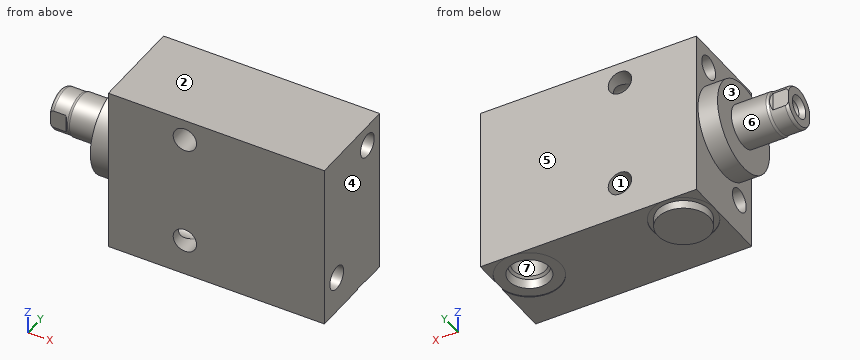
from build123d import *

# Parameters (mm, degrees)
SKETCH1_W          = 50.8
SKETCH1_H          = 28.575
EXTRUDE1_DEPTH     = 65.8368
SKETCH5_R          = 13.5001
EXTRUDE2_DEPTH     = 5.969
SKETCH6_W          = 6.35
SKETCH6_H          = 16.891
CUT_EXTRUDE4_DEPTH = 30.48
SKETCH13_R         = 7.874
EXTRUDE3_DEPTH     = 2.54
HOLE1_D            = 7.1374
HOLE1_DEPTH        = 65.8368
HOLE2_D            = 7.1374
HOLE2_DEPTH        = 28.575


with BuildPart() as part:
    # Sketch1 → Extrude1 (new body)
    with BuildSketch(Plane(origin=(0, 0, 0), x_dir=(0, 0, -1), z_dir=(1, 0, 0))):
        with Locations((2.3876, 0)):
            Rectangle(SKETCH1_W, SKETCH1_H)
    extrude(amount=EXTRUDE1_DEPTH)

    # S2D0002 → Cut-Revolve1 (revolve, cut)
    with BuildSketch(Plane(origin=(0, 4.7625, 0), x_dir=(-1, 0, 0), z_dir=(0, 1, 0)), mode=Mode.PRIVATE) as cut_revolve1_sk:
        Polygon((-15.7099, -27.5336), (-19.0499873, -27.5336), (-19.0499873, -27.7876), (-9.525, -27.7876), (-9.525, -13.5636), (-14.5034, -13.5636), (-14.5034, -24.316993135), (-15.167306865, -24.9809), align=None)
    revolve(cut_revolve1_sk.sketch.rotate(Axis((9.525, 4.7625, -19.13842003), (0, 0, 1)), 180), axis=Axis((9.525, 4.7625, -19.13842003), (0, 0, 1)), mode=Mode.SUBTRACT)  # turned: the seam where the file's is

    # Sketch3 → Cut-Revolve2 (revolve, cut)
    with BuildSketch(Plane(origin=(41.148, 4.7625, -25.146), x_dir=(1, 0, 0), z_dir=(0, 1, 0))):
        Polygon((21.5519, 2.3876), (24.8919873, 2.3876), (24.8919873, 2.6416), (15.367, 2.6416), (15.367, -11.5824), (20.3454, -11.5824), (20.3454, -0.829006865), (21.009306865, -0.1651), align=None)
    revolve(axis=Axis((56.515, 4.7625, -3.189624441), (0, 0, -1)), mode=Mode.SUBTRACT)

    # Sketch5 → Extrude2 (add)
    with BuildSketch(Plane.ZY):
        Circle(SKETCH5_R)
    extrude(amount=EXTRUDE2_DEPTH)

    # Sketch6 → Revolve1 (revolve)
    with BuildSketch(Plane(origin=(0, 0, 0), x_dir=(0, 0, 1), z_dir=(0, -1, 0)), mode=Mode.PRIVATE) as revolve1_sk:
        with Locations((-3.175, 14.4145)):
            Rectangle(SKETCH6_W, SKETCH6_H)
    revolve(revolve1_sk.sketch.rotate(Axis((5.754582971, 0, 0), (-1, 0, 0)), 180), axis=Axis((5.754582971, 0, 0), (-1, 0, 0)))  # turned: the seam where the file's is

    # S2D0001 → Cut-Revolve4 (revolve, cut)
    with BuildSketch(Plane(origin=(-18.511260017, 3.2639, 0), x_dir=(0, 1, 0), z_dir=(0, 0, 1)), mode=Mode.PRIVATE) as cut_revolve4_sk:
        Polygon((-0.7112, 2.786949769), (-0.7112, -11.653260017), (-3.2639, -13.18707692), (-3.2639, 4.348739983), (0.1905, 4.348739983), align=None)
    revolve(cut_revolve4_sk.sketch.rotate(Axis((0, 0, 0), (-1, 0, 0)), 90), axis=Axis((0, 0, 0), (-1, 0, 0)), mode=Mode.SUBTRACT)  # turned: the seam where the file's is

    # Sketch8 → Cut-Revolve5 (revolve, cut)
    with BuildSketch(Plane(origin=(0, 0, 0), x_dir=(0, 0, -1), z_dir=(0, 1, 0)), mode=Mode.PRIVATE) as cut_revolve5_sk:
        with BuildLine():
            Line((-6.35, 16.5354), (-6.096, 17.2974))
            Line((-6.096, 17.2974), (-6.096, 21.844))
            ThreePointArc((-6.096, 21.844), (-5.995678675, 22.387796865), (-5.707922533, 22.86))
            Line((-5.707922533, 22.86), (-6.35, 22.86))
            Line((-6.35, 22.86), (-6.35, 16.5354))
        make_face()
    revolve(cut_revolve5_sk.sketch.rotate(Axis((-12.65936, 0, 0), (-1, 0, 0)), 180), axis=Axis((-12.65936, 0, 0), (-1, 0, 0)), mode=Mode.SUBTRACT)  # turned: the seam where the file's is

    # Sketch12 → Cut-Extrude4 (cut, symmetric)
    with BuildSketch(Plane(origin=(0, 0, 0), x_dir=(0, -1, 0), z_dir=(0, 0, -1))):
        Polygon((5.461, 22.86), (5.461, 18.0848), (6.096, 17.4498), (6.096, 22.86), align=None)
        Polygon((-5.461, 22.86), (-5.461, 18.0848), (-6.096, 17.4498), (-6.096, 22.86), align=None)
    extrude(amount=CUT_EXTRUDE4_DEPTH, both=True, mode=Mode.SUBTRACT)

    # Sketch13 → Extrude3 (add)
    with BuildSketch(Plane(origin=(0, 0, -27.5336), x_dir=(-1, 0, 0), z_dir=(0, 0, -1))):
        with Locations((-9.525, 4.7625)):
            Circle(SKETCH13_R)
    extrude(amount=EXTRUDE3_DEPTH)

    # Hole1
    with Locations(Plane.ZY):
        with Locations((-16.6878, -7.9248), (16.6624, 7.9502)):
            Hole(HOLE1_D / 2, depth=HOLE1_DEPTH)

    # Hole2
    with Locations(Plane(origin=(0, 14.2875, 0), x_dir=(-1, 0, 0), z_dir=(0, 1, 0))):
        with Locations((-23.3172, -16.6878), (-23.3172, 16.6624)):
            Hole(HOLE2_D / 2, depth=HOLE2_DEPTH)


solid = part.part
The listing builds one solid part. Answer for the finished solid, in the listing's coordinates (mm). Face numbers are marked on the shaded views. A direction names the side the tool comes from. Coordinates: 2 decimals unless noted, no trailing zeros. Order: outer loops, then holes, each group sorted by start corner. A loop starts at its lowest first (then second) coordinate and runs counter-clockwise, first axis right, second up. Notation, with made-up numbers: M 74,-14.75 L 93,-14.75 A19 cw 93,17.25 Z; hole C -28,42 d5. An arc over 180 degrees is marked long. Use CSV: the item, a comma, the result in double quotes.
Q1. A tool of negligible diameter and unlimited length cuts with its end or side. For the marked faces 5, 6 and 7, from which of +Z, -Z, +X, -X, +Y, -Y can it reach the whole face along a straight path? Write none if from no direction.
Here are the results:
face 5,"+Z, -Z, +X, -X, +Y"
face 6,"-X"
face 7,"-Z"
Q2. Section C-C (z = 11.5) is taken. Determine the outline of the cut face in (x, y), then the cut area to 3 significant figures.
Here are the results:
outline,"M -5.97,-7.07 L 0,-7.07 L 0,-14.29 L 65.84,-14.29 L 65.84,14.29 L 0,14.29 L 0,7.07 L -5.97,7.07 Z"
area,"1,970 mm2"
Q3. Given pin 1 Ø4.5 at (x, z) = (23.32, -16.69) entering from -Y; pin 2 Ø5 at (x, y) = (-7.5, -4.5) entering from +Z; pin 3 Ø5.5 at (x, z) = (-21.5, 0.5) entering from +Y; pin 4 Ø1.5 at (y, z) = (-11, -14.5) entering from -X, each flat-ended and moving along its own axis, determine where each tip first touches the part or whether it passes through.
Here are the results:
pin 1,"through"
pin 2,"z = 13.26"
pin 3,"y = 5.46"
pin 4,"x = 0"
Q4. Straight lines are drawn through the part: L1, parallel to Z at x = 61.5, y = -7.75; L2, parallel to Z at x = 23, y = 9; L3, parallel to Z at x = 26.5, y = 9. For each, find the intervals that lie inside material, in ascending order.
Here are the results:
L1,"-27.79 to -20.25, -13.12 to 23.01"
L2,"-27.79 to -20.24, -13.13 to 13.11, 20.22 to 23.01"
L3,"-27.79 to -18.3, -15.07 to 13.25, 20.07 to 23.01"
Q5. Section B-B (x = 26) is taken. Determine the outline of the cut face in (y, z).
Here are the results:
outline,"M -14.29,-27.79 L 14.29,-27.79 L 14.29,-19.04 L -5.24,-19.04 A3.57 cw -10.61,-19.04 L -14.29,-19.04 Z; M -14.29,-14.33 L -10.61,-14.33 A3.57 cw -5.24,-14.33 L 14.29,-14.33 L 14.29,14.31 L 10.63,14.31 A3.57 cw 5.27,14.31 L -14.29,14.31 Z; M -14.29,19.02 L 5.27,19.02 A3.57 cw 10.63,19.02 L 14.29,19.02 L 14.29,23.01 L -14.29,23.01 Z"
Q6. Section D-D (x = -15) is taken. Determine the outline of the cut face in (y, z).
Here are the results:
outline,"C 0,0 d12.7; hole C 0,0 d5.11"
Q7. Determine the mould class of the marked faces 1, 2, 3 and 4 for opening direction X: pulls with the +X half, pulls with the -X half, needs draft (parallel to the pull), parting line crosses it, or undercut.
Here are the results:
face 1,"undercut"
face 2,"needs draft"
face 3,"pulls with the -X half"
face 4,"pulls with the +X half"
Q8. Section A-A (y = -9.75) is taken. Determine the outline of the cut face in (x, z).
Here are the results:
outline,"M -5.97,-9.34 L 0,-9.34 L 0,-13.62 L 21.49,-13.62 A3.57 cw 25.14,-13.62 L 65.84,-13.62 L 65.84,23.01 L 0,23.01 L 0,9.34 L -5.97,9.34 Z; M 0,-27.79 L 65.84,-27.79 L 65.84,-19.75 L 25.14,-19.75 A3.57 cw 21.49,-19.75 L 0,-19.75 Z; hole C 23.32,16.66 d7.14"
